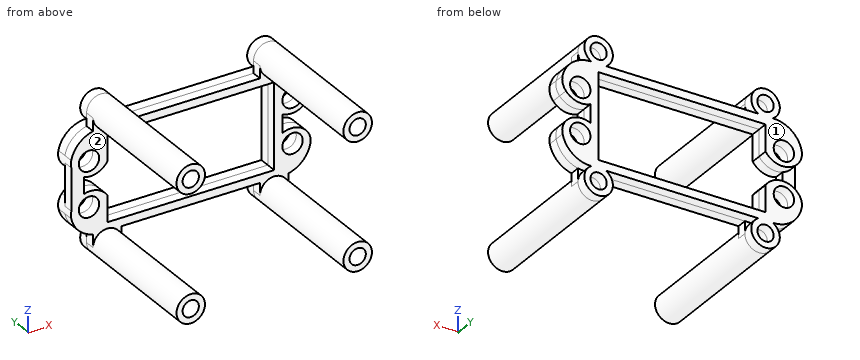
from build123d import *

# Parameters (mm, degrees)
SKETCH1_R                = 2.5
BOSS_EXTRUDE1_DEPTH      = 2.5
SKETCH4_R                = 3.5
SKETCH4_R_2              = 2
BOSS_EXTRUDE2_DEPTH      = 2.5
BOSS_EXTRUDE2_DEPTH_BACK = 35
SKETCH5_R                = 2.5
BOSS_EXTRUDE3_DEPTH      = 2.5


with BuildPart() as part:
    # Sketch1 → Boss-Extrude1 (new body)
    with BuildSketch(Plane(origin=(0, 0, 0), x_dir=(1, 0, 0), z_dir=(0, 1, 0))):
        with BuildLine():
            Line((20.5, 10.5), (-20.5, 10.5))
            Line((-20.5, 10.5), (-20.5, 4))
            ThreePointArc((-20.5, 4), (-24.40287122, 1.76806345), (-28.520566145, 3.573204173))
            ThreePointArc((-28.520566145, 3.573204173), (-29.324072849, 5.171652721), (-29.350396575, 6.960498116))
            ThreePointArc((-29.350396575, 6.960498116), (-26.904940816, 10.941842627), (-22.5, 12.5))
            Line((-22.5, 12.5), (22.5, 12.5))
            ThreePointArc((22.5, 12.5), (26.904940816, 10.941842627), (29.350396575, 6.960498116))
            ThreePointArc((29.350396575, 6.960498116), (29.324072849, 5.171652721), (28.520566145, 3.573204173))
            ThreePointArc((28.520566145, 3.573204173), (25.737402548, 1.876578025), (22.5, 2.2557411))
            Line((22.5, 2.2557411), (22.5, -2.2557411))
            ThreePointArc((22.5, -2.2557411), (25.737402548, -1.876578025), (28.520566145, -3.573204173))
            ThreePointArc((28.520566145, -3.573204173), (29.324072849, -5.171652721), (29.350396575, -6.960498116))
            ThreePointArc((29.350396575, -6.960498116), (26.904940816, -10.941842627), (22.5, -12.5))
            Line((22.5, -12.5), (-22.5, -12.5))
            ThreePointArc((-22.5, -12.5), (-26.904940816, -10.941842627), (-29.350396575, -6.960498116))
            ThreePointArc((-29.350396575, -6.960498116), (-29.324072849, -5.171652721), (-28.520566145, -3.573204173))
            ThreePointArc((-28.520566145, -3.573204173), (-24.40287122, -1.76806345), (-20.5, -4))
            Line((-20.5, -4), (-20.5, -10.5))
            Line((-20.5, -10.5), (20.5, -10.5))
            Line((20.5, -10.5), (20.5, 10.5))
        make_face()
        with Locations((-25, 5.5)):
            Circle(SKETCH1_R, mode=Mode.SUBTRACT)
        with Locations((-25, -5.5)):
            Circle(SKETCH1_R, mode=Mode.SUBTRACT)
        with Locations((25, -5.5)):
            Circle(SKETCH1_R, mode=Mode.SUBTRACT)
        with Locations((25, 5.5)):
            Circle(SKETCH1_R, mode=Mode.SUBTRACT)
    extrude(amount=BOSS_EXTRUDE1_DEPTH)

    # Sketch4 → Boss-Extrude2 (add, two sides)
    with BuildSketch(Plane(origin=(0, 0, 0), x_dir=(1, 0, 0), z_dir=(0, 1, 0))) as boss_extrude2_sk:
        with Locations((-20.5, 15.5)):
            Circle(SKETCH4_R)
        with Locations((-20.5, 15.5)):
            Circle(SKETCH4_R_2, mode=Mode.SUBTRACT)
        with Locations((20.5, 15.5)):
            Circle(SKETCH4_R)
        with Locations((20.5, 15.5)):
            Circle(SKETCH4_R_2, mode=Mode.SUBTRACT)
        with Locations((-20.5, -15.5)):
            Circle(SKETCH4_R)
        with Locations((-20.5, -15.5)):
            Circle(SKETCH4_R_2, mode=Mode.SUBTRACT)
        with Locations((20.5, -15.5)):
            Circle(SKETCH4_R)
        with Locations((20.5, -15.5)):
            Circle(SKETCH4_R_2, mode=Mode.SUBTRACT)
    extrude(amount=BOSS_EXTRUDE2_DEPTH)
    extrude(boss_extrude2_sk.sketch, amount=-BOSS_EXTRUDE2_DEPTH_BACK)

    # Sketch5 → Boss-Extrude3 (add)
    with BuildSketch(Plane(origin=(0, 0, 0), x_dir=(1, 0, 0), z_dir=(0, 1, 0))):
        with BuildLine():
            Line((-29.324072849, 5.171652721), (-29.324072849, -5.171652721))
            ThreePointArc((-29.324072849, -5.171652721), (-29.438527194, -6.064584851), (-29.350396575, -6.960498116))
            ThreePointArc((-29.350396575, -6.960498116), (-27.465923203, -10.435821373), (-24, -12.337527971))
            Line((-24, -12.337527971), (-24, -15.5))
            Line((-24, -15.5), (-22.5, -15.5))
            ThreePointArc((-22.5, -15.5), (-20.5, -13.5), (-18.5, -15.5))
            Line((-18.5, -15.5), (-17, -15.5))
            Line((-17, -15.5), (-17, -12.5))
            Line((-17, -12.5), (17, -12.5))
            Line((17, -12.5), (17, -15.5))
            Line((17, -15.5), (18.5, -15.5))
            ThreePointArc((18.5, -15.5), (20.5, -13.5), (22.5, -15.5))
            Line((22.5, -15.5), (24, -15.5))
            Line((24, -15.5), (24, -12.337527971))
            ThreePointArc((24, -12.337527971), (27.465923203, -10.435821373), (29.350396575, -6.960498116))
            ThreePointArc((29.350396575, -6.960498116), (29.324072849, -5.171652721), (28.520566145, -3.573204173))
            ThreePointArc((28.520566145, -3.573204173), (25.737402548, -1.876578025), (22.5, -2.2557411))
            Line((22.5, -2.2557411), (22.5, 2.2557411))
            ThreePointArc((22.5, 2.2557411), (25.737402548, 1.876578025), (28.520566145, 3.573204173))
            ThreePointArc((28.520566145, 3.573204173), (29.324072849, 5.171652721), (29.350396575, 6.960498116))
            ThreePointArc((29.350396575, 6.960498116), (27.465923203, 10.435821373), (24, 12.337527971))
            Line((24, 12.337527971), (24, 15.5))
            Line((24, 15.5), (22.5, 15.5))
            ThreePointArc((22.5, 15.5), (20.5, 13.5), (18.5, 15.5))
            Line((18.5, 15.5), (17, 15.5))
            Line((17, 15.5), (17, 12.5))
            Line((17, 12.5), (-17, 12.5))
            Line((-17, 12.5), (-17, 15.5))
            Line((-17, 15.5), (-18.5, 15.5))
            ThreePointArc((-18.5, 15.5), (-20.5, 13.5), (-22.5, 15.5))
            Line((-22.5, 15.5), (-24, 15.5))
            Line((-24, 15.5), (-24, 12.337527971))
            ThreePointArc((-24, 12.337527971), (-27.465923203, 10.435821373), (-29.350396575, 6.960498116))
            ThreePointArc((-29.350396575, 6.960498116), (-29.438527194, 6.064584851), (-29.324072849, 5.171652721))
        make_face()
        with Locations((-25, 5.5)):
            Circle(SKETCH5_R, mode=Mode.SUBTRACT)
        with Locations((-25, -5.5)):
            Circle(SKETCH5_R, mode=Mode.SUBTRACT)
        with Locations((25, -5.5)):
            Circle(SKETCH5_R, mode=Mode.SUBTRACT)
        with Locations((25, 5.5)):
            Circle(SKETCH5_R, mode=Mode.SUBTRACT)
        with BuildLine():
            Line((-26.208643878, 2.004095257), (-26.208643878, -2.004095257))
            ThreePointArc((-26.208643878, -2.004095257), (-23.018368657, -2.041161266), (-20.5, -4))
            Line((-20.5, -4), (-20.5, -10.5))
            Line((-20.5, -10.5), (20.5, -10.5))
            Line((20.5, -10.5), (20.5, 10.5))
            Line((20.5, 10.5), (-20.5, 10.5))
            Line((-20.5, 10.5), (-20.5, 4))
            ThreePointArc((-20.5, 4), (-23.018368657, 2.041161266), (-26.208643878, 2.004095257))
        make_face(mode=Mode.SUBTRACT)
    extrude(amount=-BOSS_EXTRUDE3_DEPTH)


solid = part.part
Could you check a few things on this model? Use its own coordinates, in mm. Face numbers are marked on the shaded views. Give positions to 0.01 mm unless a question says otherwise; leave off trailing zeros. Order: outer loops, then holes, each group sorted by start corner. A loop starts at its lowest first (then second) coordinate and runs counter-clockwise, first axis right, second up. Notation, with made-up numbers: (33, 68) -> (82, 68) arc R15 ccw to (82, 88) -> close; hole circle Ø1 at (41.25, 16.5). An arc over 180 degrees is marked (long way). Answer in a Markdown table with one row per item. Add a question column.
Item 1: Imagine slicing it at C-C (z = 0). List the corners of the cut face in (x, y) for me, and give its area (3 significant figures).
Item 2: Imagine slicing it at B-B (x = 1). List the corners of the cut face in (y, z) for me.
Item 3: Please list where these lines run through material, in increasing order: probe 1 along X at (y, z) = (1.8, 5.5); probe 2 along Z at (x, y) = (-25, 1.8); probe 3 along X at (y, z) = (-0.5, -3.5).
Item 4: Imagine slicing it at A-A (y = -7). List the corners of the cut face in (x, z) for me.
Item 5: Imagine slicing it at D-D (x = -25). List the corners of the cut face in (y, z) for me, and give its area (3 significant figures).
Item 6: We'd pull the mould along Z, two halves only. Please class the marked faces 1 and 2: pulls with the +Z half, pulls with the -Z half, needs draft (parallel to the pull), parting line crosses it, or undercut.
Item 7: I'm going to push flat-ended pins straight in: P1, Ø2.5, axis at x = -28.5, z = 1, coming from the +Y side; P2, Ø2, axis at x = 5, y = -1.5, coming from the -Z side; P3, Ø0.8, axis at y = -1.5, z = -13.5, coming from the +X side. Where does each tip first touch, or does it pass through?
Result:
| question | item | result |
|---|---|---|
| 1 | outline | (-29.32, -2.5) -> (-26.21, -2.5) -> (-26.21, 0) -> (-29.32, 0) -> close; (20.5, -2.5) -> (22.5, -2.5) -> (22.5, 2.5) -> (20.5, 2.5) -> close |
| 1 | area | 17.8 mm2 |
| 2 | outline | (-2.5, -12.5) -> (2.5, -12.5) -> (2.5, -10.5) -> (-2.5, -10.5) -> close; (-2.5, 10.5) -> (2.5, 10.5) -> (2.5, 12.5) -> (-2.5, 12.5) -> close |
| 3 | probe 1 | -29.39 to -27.5, -22.5 to -20.5, 20.5 to 22.5, 27.5 to 29.39 |
| 3 | probe 2 | -12.04 to -8, -3 to -1.77, 1.77 to 3, 8 to 12.04 |
| 3 | probe 3 | -29.32 to -26.5, -23.5 to -20.88, 20.5 to 23.5, 26.5 to 28.46 |
| 4 | outline | circle Ø7 at (-20.5, -15.5); circle Ø7 at (-20.5, 15.5); circle Ø7 at (20.5, -15.5); circle Ø7 at (20.5, 15.5); hole circle Ø4 at (-20.5, -15.5); hole circle Ø4 at (-20.5, 15.5); hole circle Ø4 at (20.5, -15.5); hole circle Ø4 at (20.5, 15.5) |
| 5 | outline | (-2.5, -12.04) -> (2.5, -12.04) -> (2.5, -8) -> (-2.5, -8) -> close; (-2.5, -3) -> (2.5, -3) -> (2.5, -1.77) -> (-2.5, -1.77) -> close; (-2.5, 1.77) -> (2.5, 1.77) -> (2.5, 3) -> (-2.5, 3) -> close; (-2.5, 8) -> (2.5, 8) -> (2.5, 12.04) -> (-2.5, 12.04) -> close |
| 5 | area | 52.7 mm2 |
| 6 | face 1 | needs draft |
| 6 | face 2 | undercut |
| 7 | P1 | y = 0 |
| 7 | P2 | z = -12.5 |
| 7 | P3 | x = 24 |
